```python
from build123d import *

# Parameters (mm, degrees)
F0_W     = 25
F0_H     = 32
F1_DEPTH = 3.75
F2_W     = 12.2002800852
F2_H     = 18
F3_DEPTH = 3.75
F4_R     = 1.5
F5_DEPTH = 32
F6_R     = 3
F7_R     = 1.5
F8_DEPTH = 3.75


with BuildPart() as f1:
    # F0 (on Top) → F1 (new body, symmetric)
    with BuildSketch(Plane.XY):
        with Locations((12.5, 16)):
            Rectangle(F0_W, F0_H)
    extrude(amount=F1_DEPTH, both=True)

    # F2 (on Top) → F3 (cut, symmetric)
    with BuildSketch(Plane.XY):
        with Locations((23.1001400426, 16)):
            Rectangle(F2_W, F2_H)
    extrude(amount=F3_DEPTH, both=True, mode=Mode.SUBTRACT)

    # F4 (on Front) → F5 (cut)
    with BuildSketch(Plane.XZ):
        with Locations((21, 0)):
            Circle(F4_R)
    extrude(amount=-F5_DEPTH, mode=Mode.SUBTRACT)

    # F6
    f6_edges = [f1.edges().sort_by_distance(p)[0] for p in [
        (25, 28.5, -3.75),
        (25, 28.5, 3.75),
        (25, 3.5, 3.75),
        (25, 3.5, -3.75),
    ]]
    fillet(f6_edges, radius=F6_R)

    # F7 (on Top) → F8 (cut, symmetric)
    with BuildSketch(Plane.XY):
        with Locations((12.5, 3.5)):
            Circle(F7_R)
        with Locations((12.5, 28.5)):
            Circle(F7_R)
    extrude(amount=F8_DEPTH, both=True, mode=Mode.SUBTRACT)

    # F9: F1 across plane


with BuildPart() as f1_1:
    add(f1.part)
    add(f1.part.mirror(Plane.YZ))


solid = f1_1.part
```
For this review, take the finished solid that the model builds, in its own axes (mm). A direction names the side the tool comes from. Coordinates: 2 decimals unless noted, no trailing zeros. Loops run counter-clockwise (first coordinate to the right, second up) from the corner with the lowest first, then second, coordinate; pieces in that order, holes last.
1. Add section B-B, the plane z = 0. Count the separate pieces of the cut face and the enclosed holes in it, then the cut area to 3 significant figures.
2. Add section A-A, the plane y = 3.5. Give the boundary of the cut face in (x, z), then the cut area to 3 significant figures.
3. For line 1 (Y direction, x = 12.5, z = -1); line 2 (Y direction, x = -21, z = -2.75); line 3 (Y direction, x = -11.5, z = -0.5), list the stretches that pass through material, from the lowest coordinate up.
4. Add section C-C, the plane x = -12.5. Give the boundary of the cut face in (y, z).
5. For faces 5 (the cylindrical face through (19.5, 28.45, 0.07)), 6 (the flat face through (-19, 25, 0)), 7 (the flat face through (19, 25, 0)), list the 3-axis set-ups (+Z, -Z, +X, -X, +Y, -Y) from which the entire face can be reached by the end or side of a thin tool; tool diameter is ignored.
6. Insertion check: P1, Ø2.5, axis at x = -21, z = 0, coming from the -Y side; P2, Ø2, axis at y = 12, z = -1, coming from the -X side; P3, Ø4, axis at y = 17.5, z = -0.5, coming from the +X side. Each pin has a flat end and moves straight along its axis. Give the tip position at first contact, or say it passes through.
7. Add section D-D, the plane x = 21. Give the boundary of the cut face in (y, z), then the cut area to 3 significant figures.
8. Mouldability with a two-part tool opening along Z and no side actions: class faces 1 (the cylindrical face through (-19.5, 3.45, 0.07)), 2 (the cylindrical face through (24.1, 28.55, 2.89)), 3 (the flat face through (-17, 16, 0)), 4 (the cylindrical face through (19.5, 3.45, 0.07)) as +Z half, -Z half, draft (parallel to the pull), parting line (faces both ways), or undercut.
Result:
1. separate pieces: 5
1. enclosed holes: 4
1. area: 1,200 mm2
2. outline: (-25, -0.75) arc R3 ccw to (-22, -3.75) - (-14, -3.75) - (-14, 3.75) - (-22, 3.75) arc R3 ccw to (-25, 0.75) - close; (-11, -3.75) - (11, -3.75) - (11, 3.75) - (-11, 3.75) - close; (14, -3.75) - (22, -3.75) arc R3 ccw to (25, -0.75) - (25, 0.75) arc R3 ccw to (22, 3.75) - (14, 3.75) - close; hole circle Ø3 at (-21, 0); hole circle Ø3 at (21, 0)
2. area: 308 mm2
3. line 1: y = 0 to 2, 5 to 27, 30 to 32
3. line 2: y = 0 to 7, 25 to 32
3. line 3: y = 0 to 2.38, 4.62 to 27.38, 29.62 to 32
4. outline: (0, -3.75) - (2, -3.75) - (2, 3.75) - (0, 3.75) - close; (5, -3.75) - (27, -3.75) - (27, 3.75) - (5, 3.75) - close; (30, -3.75) - (32, -3.75) - (32, 3.75) - (30, 3.75) - close
5. face 5: +Y, -Y
5. face 6: +Z, -Z, -X
5. face 7: +Z, -Z, +X
6. P1: passes through
6. P2: stops at x = -17
6. P3: stops at x = 17
7. outline: (0, -3.75) - (7, -3.75) - (7, -1.5) - (0, -1.5) - close; (0, 1.5) - (7, 1.5) - (7, 3.75) - (0, 3.75) - close; (25, -3.75) - (32, -3.75) - (32, -1.5) - (25, -1.5) - close; (25, 1.5) - (32, 1.5) - (32, 3.75) - (25, 3.75) - close
7. area: 63.0 mm2
8. face 1: undercut
8. face 2: +Z half
8. face 3: draft
8. face 4: undercut
